```python
from build123d import *

# Parameters (mm, degrees)
ESQUISSE1_R             = 1.15
BOSS_EXTRU_1_DEPTH      = 1.15
CONG_1_R                = 0.5
ESQUISSE2_W             = 20
ESQUISSE2_H             = 31.4
BOSS_EXTRU_2_DEPTH      = 6.3
ESQUISSE4_W             = 6.5
ESQUISSE4_H             = 3
ENL_V_MAT_EXTRU_1_DEPTH = 0.1


with BuildPart() as part:
    # Esquisse1 → Boss.-Extru.1 (new body)
    with BuildSketch(Plane(origin=(0, 0, 0), x_dir=(1, 0, 0), z_dir=(0, 1, 0))):
        Polygon((-2.55, -19.65), (-2.55, -20.75), (2.55, -20.75), (2.55, -19.65), (8.35, -19.65), (8.35, 19.65), (2.55, 19.65), (2.55, 20.75), (-2.55, 20.75), (-2.55, 19.65), (-8.35, 19.65), (-8.35, -19.65), align=None)
        with Locations(Location((0, -17.75, 0), (0, 0, 270))):
            Circle(ESQUISSE1_R, mode=Mode.SUBTRACT)
        with Locations(Location((0, 17.75, 0), (0, 0, 270))):
            Circle(ESQUISSE1_R, mode=Mode.SUBTRACT)
    extrude(amount=BOSS_EXTRU_1_DEPTH)

    # Congé1
    cong_1_edges = [part.edges().sort_by_distance(p)[0] for p in [
        (-2.55, 0.575, 19.65),
        (-2.55, 0.575, -19.65),
        (2.55, 0.575, -19.65),
        (2.55, 0.575, 19.65),
    ]]
    fillet(cong_1_edges, radius=CONG_1_R)

    # Esquisse2 → Boss.-Extru.2 (add)
    with BuildSketch(Plane(origin=(0, 1.15, 0), x_dir=(1, 0, 0), z_dir=(0, 1, 0))):
        Rectangle(ESQUISSE2_W, ESQUISSE2_H)
    extrude(amount=BOSS_EXTRU_2_DEPTH)

    # Esquisse4 → Enlèv. mat.-Extru.1 (cut)
    with BuildSketch(Plane(origin=(0, 7.45, 0), x_dir=(1, 0, 0), z_dir=(0, 1, 0))):
        Polygon((0, 12.9), (0, 10.5), (4.8, 10.5), (4.8, -10.1), (2.5, -10.1), (2.5, -11.3), (6, -11.3), (6, 11.7), (2.5, 11.7), (2.5, 12.9), align=None)
        Polygon((-2.5, -11.3), (-2.5, -10.1), (-4.8, -10.1), (-4.8, 10.5), (0, 10.5), (0, 12.9), (-2.5, 12.9), (-2.5, 11.7), (-6, 11.7), (-6, -11.3), align=None)
        with Locations((0, 7.7)):
            Rectangle(ESQUISSE4_W, ESQUISSE4_H)
        with Locations((0, -2.3)):
            Rectangle(ESQUISSE4_W, ESQUISSE4_H)
        with Locations((0, -7.3)):
            Rectangle(ESQUISSE4_W, ESQUISSE4_H)
        with Locations((0, 2.7)):
            Rectangle(ESQUISSE4_W, ESQUISSE4_H)
    extrude(amount=-ENL_V_MAT_EXTRU_1_DEPTH, mode=Mode.SUBTRACT)


solid = part.part
```
The listing builds one solid part. Answer for the finished solid, in the listing's coordinates (mm). A direction names the side the tool comes from. Coordinates: 2 decimals unless noted, no trailing zeros. Loops run counter-clockwise (first coordinate to the right, second up) from the corner with the lowest first, then second, coordinate; pieces in that order, holes last. Notation, with made-up numbers: (52, 61.25) - (99, 61.25) arc R24 ccw to (99, 72.25) - close; hole circle Ø11 at (5.25, -16.5). An arc over 180 degrees is marked (long way). Use a Markdown table: item, result. Add a question column.
1) Find the intervals of material crossed by line 1 (X direction, y = 0.9, z = 17.75); line 2 (Z direction, x = 2, y = 5.5); line 3 (Y direction, x = -8.5, z = 13), in increasing order.
2) The part is cut by section A-A, the plane z = -17.75. Give the vertices of the cut face in (x, y), and give its area (3 significant figures).
3) Given pin 1 (2.5 mm diameter, centred on x = -1, z = -19, fed in from +Y); pin 2 (3 mm diameter, centred on x = 3.5, y = 3.5, fed in from +Z); pin 3 (3 mm diameter, centred on x = -4, y = 6.5, fed in from -Z), each flat-ended and moving along its own axis, determine where each tip first touches the part or whether it passes through.
4) The part is cut by section C-C, the plane z = -2.5. Give the vertices of the cut face in (x, y).
5) For faces 5 (the flat face through (-8.35, 0.6, -0.3)), 6 (the flat face through (-5.7, 0.6, -19.65)), 7 (the flat face through (-0.1, 1.15, 19.3)), determine the directions among +Z, -Z, +X, -X, +Y, -Y from which every point of the face is accessible in a straight line to the end or side of a thin tool.
6) The part is cut by section B-B, the plane x = -7.5. Give the vertices of the cut face in (y, z).
7) The part is cut by section D-D, the plane y = 4.75. Give the vertices of the cut face in (x, z).
8) The mould has two halves that part along Z. Classify faces 1 (the flat face through (0, 4, 15.7)), 2 (the flat face through (0, 7.35, 7)), 3 (the flat face through (0, 0.6, -20.75)), 4 (the flat face through (0, 7.35, -8)): released by +Z, released by -Z, zero draft, split by the parting line, or undercut.
Here are the results:
| question | item | result |
|---|---|---|
| 1 | line 1 | x = -8.35 to -1.15, 1.15 to 8.35 |
| 1 | line 2 | z = -15.7 to 15.7 |
| 1 | line 3 | y = 1.15 to 7.45 |
| 2 | outline | (-8.35, 0) - (-1.15, 0) - (-1.15, 1.15) - (-8.35, 1.15) - close; (1.15, 0) - (8.35, 0) - (8.35, 1.15) - (1.15, 1.15) - close |
| 2 | area | 16.6 mm^2 |
| 3 | pin 1 | stops at y = 1.15 |
| 3 | pin 2 | stops at z = 15.7 |
| 3 | pin 3 | stops at z = -15.7 |
| 4 | outline | (-10, 1.15) - (-8.35, 1.15) - (-8.35, 0) - (8.35, 0) - (8.35, 1.15) - (10, 1.15) - (10, 7.45) - (6, 7.45) - (6, 7.35) - (4.8, 7.35) - (4.8, 7.45) - (3.25, 7.45) - (3.25, 7.35) - (-3.25, 7.35) - (-3.25, 7.45) - (-4.8, 7.45) - (-4.8, 7.35) - (-6, 7.35) - (-6, 7.45) - (-10, 7.45) - close |
| 5 | face 5 | +Z, -Z, -X, -Y |
| 5 | face 6 | -Z, -X, +Y, -Y |
| 5 | face 7 | +Z, +X, -X, +Y |
| 6 | outline | (0, -19.65) - (1.15, -19.65) - (1.15, -15.7) - (7.45, -15.7) - (7.45, 15.7) - (1.15, 15.7) - (1.15, 19.65) - (0, 19.65) - close |
| 7 | outline | (-10, -15.7) - (10, -15.7) - (10, 15.7) - (-10, 15.7) - close |
| 8 | face 1 | released by +Z |
| 8 | face 2 | undercut |
| 8 | face 3 | released by -Z |
| 8 | face 4 | undercut |
